```python
from build123d import *

# Parameters (mm, degrees)
BOSS_EXTRUDE1_DEPTH = 30
SKETCH2_W           = 2.5
SKETCH2_H           = 17.424704808
BOSS_EXTRUDE2_DEPTH = 5
CHAMFER1_SIZE       = 1.25
SKETCH3_W           = 2.5
SKETCH3_H           = 15
BOSS_EXTRUDE3_DEPTH = 5
CHAMFER2_SIZE       = 1.25
FILLET1_R           = 5


with BuildPart() as part:
    # Sketch1 → Boss-Extrude1 (new body)
    with BuildSketch(Plane(origin=(0, 0, 0), x_dir=(1, 0, 0), z_dir=(0, 1, 0))):
        Polygon((0, 0), (105, 0), (105, 80), (100, 80), (100, 5), (0, 5), align=None)
    extrude(amount=BOSS_EXTRUDE1_DEPTH)

    # Sketch2 → Boss-Extrude2 (add)
    with BuildSketch(Plane.ZY):
        with Locations((-3.75, 15)):
            Rectangle(SKETCH2_W, SKETCH2_H)
    extrude(amount=BOSS_EXTRUDE2_DEPTH)

    # Chamfer1
    chamfer1_edges = [part.edges().sort_by_distance(p)[0] for p in [
        (-5, 15, -5),
    ]]
    chamfer(chamfer1_edges, length=CHAMFER1_SIZE)

    # Sketch3 → Boss-Extrude3 (add)
    with BuildSketch(Plane(origin=(0, 0, -80), x_dir=(-1, 0, 0), z_dir=(0, 0, -1))):
        with Locations((-101.25, 15)):
            Rectangle(SKETCH3_W, SKETCH3_H)
    extrude(amount=BOSS_EXTRUDE3_DEPTH)

    # Chamfer2
    chamfer2_edges = [part.edges().sort_by_distance(p)[0] for p in [
        (100, 15, -85),
    ]]
    chamfer(chamfer2_edges, length=CHAMFER2_SIZE)

    # Fillet1
    fillet1_edges = [part.edges().sort_by_distance(p)[0] for p in [
        (105, 15, 0),
    ]]
    fillet(fillet1_edges, radius=FILLET1_R)


solid = part.part
```
The listing builds one solid part. Answer for the finished solid, in the listing's coordinates (mm). A direction names the side the tool comes from. Coordinates: 2 decimals unless noted, no trailing zeros. Write each loop counter-clockwise with the first axis right and the second up, starting at its lowest first coordinate (ties: lowest second). Pieces come first, ordered by that corner, then holes. Notation, with made-up numbers: (76.25, 51) - (115.25, 51) arc R24 cw to (115.25, 88) - close; hole circle Ø9 at (79.25, -7.75). An arc over 180 degrees is marked (long way). One line per item, written item: value.
1) Find section A-A (y = 13). Give the vertices of the cut face in (x, z).
Geometry check:
outline: (-5, -3.75) - (-3.75, -5) - (100, -5) - (100, -83.75) - (101.25, -85) - (102.5, -85) - (102.5, -80) - (105, -80) - (105, -5) arc R5 ccw to (100, 0) - (0, 0) - (0, -2.5) - (-5, -2.5) - close
2) Each of these flat-tipped pins is pushed along its axis until it touches: pin 1 Ø2 at (y, z) = (26, -62) entering from -X; pin 2 Ø1.2 at (x, z) = (-2, -4.5) entering from -Y; pin 3 Ø1.5 at (x, y) = (13.5, 16.5) entering from -Z. Where does it stop, or does it pass through?
Geometry check:
pin 1: stops at x = 100
pin 2: stops at y = 6.29
pin 3: stops at z = -5
3) A tool of negligible diameter and unlimited length cuts with its end or side. For faces 1 (the flat face through (102.5, 15, -82)), 2 (the flat face through (101, 22.5, -82)), 3 (the flat face through (-2, 15, -2.5)), 4 (the flat face through (49, 15, -5)), from which of +Z, -Z, +X, -X, +Y, -Y can it reach the whole face along a straight path? Write none if from no direction.
Geometry check:
face 1: -Z, +X, +Y, -Y
face 2: -Z, +X, -X, +Y
face 3: +Z, -X, +Y, -Y
face 4: -Z, -X, +Y, -Y
4) Consider line 1 along Z through (x, y) = (33, 16.75); line 2 along X through (y, z) = (25.5, -5.5); line 3 along X through (y, z) = (4.75, -3.5). Determine where each line is inside the solid, lowest interval first. Write a range as from..to.
Geometry check:
line 1: z = -5..0
line 2: x = 100..105
line 3: x = 0..104.77
5) Find section D-D (x = 42.5). Give the vertices of the cut face in (y, z).
Geometry check:
outline: (0, -5) - (30, -5) - (30, 0) - (0, 0) - close
6) Find section C-C (y = 2.5). Give the vertices of the cut face in (x, z), and give its area (3 significant figures).
Geometry check:
outline: (0, -5) - (100, -5) - (100, -80) - (105, -80) - (105, -5) arc R5 ccw to (100, 0) - (0, 0) - close
area: 895 mm2
7) Find section B-B (z = -22). Give the vertices of the cut face in (x, y), and give its area (3 significant figures).
Geometry check:
outline: (100, 0) - (105, 0) - (105, 30) - (100, 30) - close
area: 150 mm2
